For this review, use the dimensioned drawing (mm, ordinates from the lowest corner) and the shaded views. Round coordinates to 2 decimals unless told otherwise and drop trailing zeros. Loops run counter-clockwise (first coordinate to the right, second up) from the corner with the lowest first, then second, coordinate; pieces in that order, holes last. Notation, with made-up numbers: (24.25, 57) -> (49.25, 57) arc R14 ccw to (49.25, 61) -> close; hole circle Ø5 at (31.25, 28.25). An arc over 180 degrees is marked (long way). Write each question's results on one line, items separated by ' | '. Start each with the question number.
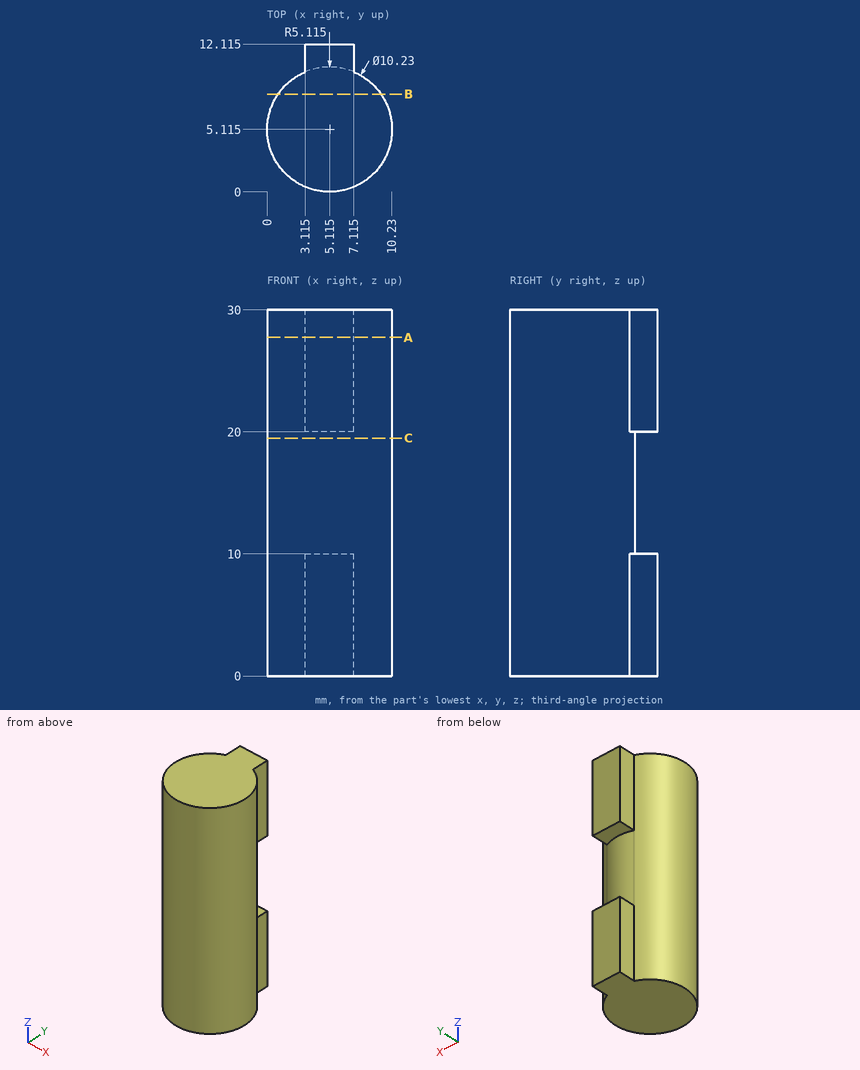
1) Take a section at B-B (y = 8). Write out the cut boundary in (x, z), plus the area to 3 significant figures.
2) Take a section at C-C (z = 19.5). Write out the cut boundary in (x, y) (3 decimals), plus the area to 3 significant figures.
3) To check wall thickness, follow line 1 (X direction, y = 5, z = 21); line 2 (X direction, y = 11.5, z = 4.75) (3 decimals); line 3 (Y direction, x = 2, z = 11). State the ranges of each line that lie inside material, in increasing order. Write a range as from..to.
4) Take a section at A-A (z = 27.75). Write out the cut boundary in (x, y) (3 decimals), plus the area to 3 significant figures.
5) Insertion check: pin 1 (1.8 mm diameter, centred on y = 11.5, z = 7.5, fed in from -X) (3 decimals); pin 2 (2 mm diameter, centred on x = 5.5, z = 13, fed in from +Y); pin 3 (2.5 mm diameter, centred on y = 11.5, z = 25.5, fed in from +X) (3 decimals). Each pin has a flat end and moves straight along its axis. Give the tip position at first contact, or say it passes through.
Geometry check:
1) outline: (0.89, 0) -> (9.34, 0) -> (9.34, 30) -> (0.89, 30) -> close | area: 253 mm^2
2) outline: circle Ø10.23 at (5.115, 5.115) | area: 82.2 mm^2
3) line 1: x = 0..10.23 | line 2: x = 3.115..7.115 | line 3: y = 1.06..9.17
4) outline: (3.115, 9.823) arc R5.115 ccw (long way) to (7.115, 9.823) -> (7.115, 12.115) -> (3.115, 12.115) -> close | area: 90.3 mm^2
5) pin 1: stops at x = 3.115 | pin 2: stops at y = 10.23 | pin 3: stops at x = 7.115
